Check sheet for the modelled part. Datum: model origin and axes. Units: mm. Face numbers are marked on the shaded views. A direction names the side the tool comes from. Give positions to 0.01 mm unless a question says otherwise; leave off trailing zeros. Write each loop counter-clockwise with the first axis right and the second up, starting at its lowest first coordinate (ties: lowest second). Pieces come first, ordered by that corner, then holes. Notation, with made-up numbers: M 32,17 L 73,17 A11 cw 73,35 Z; hole C 4,42 d3. An arc over 180 degrees is marked long. Write item = value, one per line. Start each with the question number.
1) Scan lines: line 1 along Y through (x, z) = (-62.4, -48.95); line 2 along Z through (x, y) = (-12, 64); line 3 along Z through (x, y) = (5.5, 45.5). Record each from-to range of solid material in increasing order. Write a range as [from, to].
2) Cross-section at D-D, the plane z = -36. Record the cut outline in (x, y), plus the area to 3 significant figures.
3) Cross-section at A-A, the plane x = -62.4. Record the cut outline in (y, z), plus the area to 3 significant figures.
4) Go/stop test with flat-tipped pins: pin 1 (8 mm diameter, centred on x = -46, z = -37.5, fed in from -Y); pin 2 (12 mm diameter, centred on x = -29.5, y = 101.5, fed in from -Z); pin 3 (12 mm diameter, centred on x = -18, z = -11.5, fed in from +Y). Record where each tip stops, or that it passes through.
5) Cross-section at B-B, the plane y = -4.6. Record the cut outline in (x, z).
6) Access from +Z, -Z, +X, -X, +Y, -Y to the whole of each face (thin tool, end or side, straight path). Record for the marked faces 1, 2, 3, 4 and 5.
7) Cross-section at C-C, the plane z = -48.5. Record the cut outline in (x, y), plus the area to 3 significant figures.
```python
from build123d import *

# Parameters (mm, degrees)
SKETCH_1_W      = 40
SKETCH_1_H      = 116
PAD_DEPTH       = 5
PAD001_DEPTH    = 5
PAD002_DEPTH    = 126.2
SKETCH005_W     = 9.2
SKETCH005_H     = 9.2
POCKET_DEPTH    = 33.001
PAD004_DEPTH    = 2
PAD005_DEPTH    = 51
SKETCH006_W     = 2
SKETCH006_H     = 117
PAD006_DEPTH    = 23
PAD007_DEPTH    = 2
PAD008_DEPTH    = 9.2
SKETCH009_W     = 9.2
SKETCH009_H     = 5
PAD009_DEPTH    = 9.2
SKETCH010_R     = 1.6
POCKET001_DEPTH = 5
SKETCH011_W     = 107.6
SKETCH011_H     = 1.4
PAD010_DEPTH    = 10
SKETCH012_W     = 18.1
SKETCH012_H     = 2.08
POCKET002_DEPTH = 11
CHAMFER_SIZE    = 2
PAD011_DEPTH    = 51


with BuildPart() as part:
    # Sketch_1 → Pad (new body)
    with BuildSketch(Plane.XY):
        with Locations((-20, 58)):
            Rectangle(SKETCH_1_W, SKETCH_1_H)
    extrude(amount=PAD_DEPTH)

    # Sketch → Pad001 (join)
    with BuildSketch(Plane.XY):
        Polygon((0, 0), (-40, 0), (-40, -10.2), (-27.222153, -10.2), (0, -15), align=None)
    extrude(amount=PAD001_DEPTH)

    # Sketch001 (on Face6 of Pad001) → Pad002 (join)
    with BuildSketch(Plane.XZ.offset(10.2)):
        Polygon((-40, 5), (-68, -23), (-68, -28), (-66, -28), (-66, -26), (-40, 0), align=None)
    extrude(amount=-PAD002_DEPTH)

    # Sketch005 (on Face13 of Pad002) → Pocket (cut, through all)
    with BuildSketch(Plane.XY.offset(5)):
        with Locations((-63.4, -5.6)):
            Rectangle(SKETCH005_W, SKETCH005_H)
    extrude(amount=-POCKET_DEPTH, mode=Mode.SUBTRACT)

    # Sketch003 → Pad004 (join)
    with BuildSketch(Plane.XZ.offset(10.2)):
        Polygon((-58.8, -51), (-58.8, -18.8), (-40, 0), (-27.222153, 0), (-27.222153, -51), align=None)
    extrude(amount=-PAD004_DEPTH)

    # Sketch004 (on Face12 of Pad004) → Pad005 (join)
    with BuildSketch(Plane(origin=(0, 0, 0), x_dir=(1, 0, 0), z_dir=(0, 0, -1))):
        Polygon((-27.222153, 10.2), (0, 15), (0, 13), (-27.222153, 8.2), align=None)
    extrude(amount=PAD005_DEPTH)

    # Sketch006 (on Face8 of Pad005) → Pad006 (join)
    with BuildSketch(Plane(origin=(0, 0, -28), x_dir=(1, 0, 0), z_dir=(0, 0, -1))):
        with Locations((-67, -57.5)):
            Rectangle(SKETCH006_W, SKETCH006_H)
    extrude(amount=PAD006_DEPTH)

    # Sketch007 (on Face27 of Pad006) → Pad007 (join)
    with BuildSketch(Plane.XZ.offset(1)):
        Polygon((-58.8, -18.8), (-66, -26), (-66, -53), (-58.8, -53), align=None)
    extrude(amount=-PAD007_DEPTH)

    # Sketch008 (on Face22 of Pad007) → Pad008 (join)
    with BuildSketch(Plane(origin=(0, -8.2, 0), x_dir=(-1, 0, 0), z_dir=(0, 1, 0))):
        Polygon((56.8, -16.8), (56.8, -53), (58.8, -53), (58.8, -18.8), align=None)
    extrude(amount=PAD008_DEPTH)

    # Sketch009 (on Face32 of Pad008) → Pad009 (join)
    with BuildSketch(Plane.XZ.offset(1)):
        with Locations((-63.4, -48.5)):
            Rectangle(SKETCH009_W, SKETCH009_H)
    extrude(amount=PAD009_DEPTH)

    # Sketch010 (on Face43 of Pad009) → Pocket001 (cut)
    with BuildSketch(Plane.XY.offset(-46)):
        with Locations((-62.4, -4.6)):
            Circle(SKETCH010_R)
    extrude(amount=-POCKET001_DEPTH, mode=Mode.SUBTRACT)

    # Sketch011 (on Face3 of Pocket001) → Pad010 (join)
    with BuildSketch(Plane.YZ):
        with Locations((41, 2.64)):
            Rectangle(SKETCH011_W, SKETCH011_H)
    extrude(amount=PAD010_DEPTH)

    # Sketch012 (on Face1 of Pad010) → Pocket002 (cut)
    with BuildSketch(Plane(origin=(0, 116, 0), x_dir=(-1, 0, 0), z_dir=(0, 1, 0))):
        with Locations((20, 2.54)):
            Rectangle(SKETCH012_W, SKETCH012_H)
    extrude(amount=-POCKET002_DEPTH, mode=Mode.SUBTRACT)

    # Chamfer
    chamfer_edges = [part.edges().sort_by_distance(p)[0] for p in [
        (-13.611076, -12.6, 5),
        (-33.611076, -10.2, 5),
    ]]
    chamfer(chamfer_edges, length=CHAMFER_SIZE)

    # Sketch013 (on Face32 of Chamfer) → Pad011 (join)
    with BuildSketch(Plane(origin=(0, 0, 0), x_dir=(1, 0, 0), z_dir=(0, 0, -1))):
        Polygon((-5.671282, 12), (1.5, 12), (1.5, 13), (0, 13), align=None)
    extrude(amount=PAD011_DEPTH)


solid = part.part
```
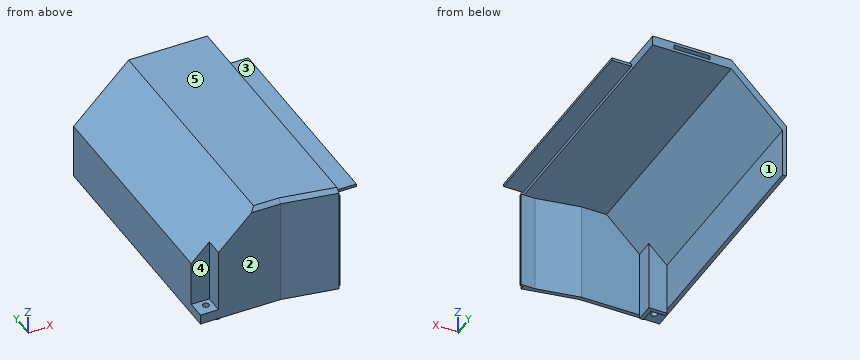
Reply:
q1.line_1 = [-10.2, -6.2], [-3, 1]
q1.line_2 = [0, 5]
q1.line_3 = [1.94, 3.34]
q2.outline = M -68,-1 L -58.8,-1 L -58.8,-10.2 L -27.22,-10.2 L 0,-15 L 0,-13 L 1.5,-13 L 1.5,-12 L -5.67,-12 L -27.22,-8.2 L -56.8,-8.2 L -56.8,1 L -66,1 L -66,116 L -68,116 Z
q2.area = 389 mm2
q3.outline = M -10.2,-51 L -6.2,-51 L -6.2,-46 L -10.2,-46 Z; M -3,-51 L -1,-51 L -1,-53 L 1,-53 L 1,-22.4 L 116,-22.4 L 116,-17.4 L -1,-17.4 L -1,-46 L -3,-46 Z
q3.area = 676 mm2
q4.pin_1 = -10.2
q4.pin_2 = 0
q4.pin_3 = -8.77
q5.outline = M -68,-51 L -64,-51 L -64,-46 L -68,-46 Z; M -60.8,-51 L -58.8,-51 L -58.8,-53 L -56.8,-53 L -56.8,-16.8 L -40,0 L 0,0 L 0,1.94 L 10,1.94 L 10,3.34 L 0,3.34 L 0,5 L -40,5 L -58.8,-13.8 L -58.8,-46 L -60.8,-46 Z
q6.face_1 = -Z, +X, +Y
q6.face_2 = +Z, -Z, -X, -Y
q6.face_3 = +Z, +X, +Y, -Y
q6.face_4 = +Z, -X, -Y
q6.face_5 = +Z, +X, -X, +Y, -Y
q7.outline = M -68,-10.2 L -27.22,-10.2 L 0,-15 L 0,-13 L 1.5,-13 L 1.5,-12 L -5.67,-12 L -27.22,-8.2 L -56.8,-8.2 L -56.8,1 L -66,1 L -66,116 L -68,116 Z; hole C -62.4,-4.6 d3.2
q7.area = 465 mm2
